For this review, take the finished solid that the model builds, in its own axes (mm). Face numbers are marked on the shaded views. A direction names the side the tool comes from. Round coordinates to 2 decimals unless told otherwise and drop trailing zeros. Order: outer loops, then holes, each group sorted by start corner. A loop starts at its lowest first (then second) coordinate and runs counter-clockwise, first axis right, second up. Notation, with made-up numbers: M 85.25,-34 L 131.25,-34 A22 cw 131.25,-19 Z; hole C 75.5,-4 d2. An arc over 180 degrees is marked long. Put each result on its own line as item: value.
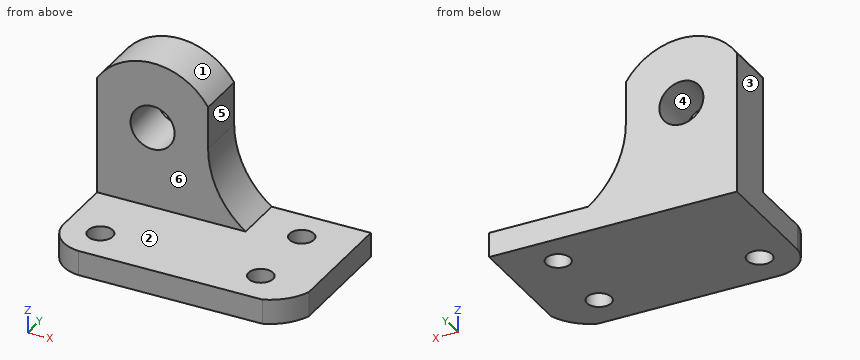
from build123d import *

# Parameters (mm, degrees)
F0_W      = 63.5
F0_H      = 38.1
F1_DEPTH  = 6.35
F3_DEPTH  = 25.4
F4_W      = 38.1
F4_H      = 12.7
F5_DEPTH  = 38.1
F7_DEPTH  = 25.4
F8_R      = 5.646791
F9_DEPTH  = 25.4
F10_R     = 3.186215
F10_R_2   = 3.13512
F10_R_3   = 3.110599
F11_DEPTH = 25.4


with BuildPart() as f1:
    # F0 (on Top) → F1 (new body)
    with BuildSketch(Plane.XY):
        with Locations((31.75, 19.05)):
            Rectangle(F0_W, F0_H)
    extrude(amount=F1_DEPTH)

    # F2 (on face) → F3 (cut)
    with BuildSketch(Plane.XY.offset(6.35)):
        with BuildLine():
            ThreePointArc((8.66646, 0), (2.760987, 2.655022), (0, 8.511703))
            Line((0, 8.511703), (0, 0))
            Line((0, 0), (8.66646, 0))
        make_face()
        with BuildLine():
            ThreePointArc((63.5, 7.892669), (60.506344, 3.058511), (55.712957, 0))
            Line((55.712957, 0), (63.5, 0))
            Line((63.5, 0), (63.5, 7.892669))
        make_face()
    extrude(amount=-F3_DEPTH, mode=Mode.SUBTRACT)

    # F4 (on face) → F5 (join)
    with BuildSketch(Plane.XY.offset(6.35)):
        with Locations((19.05, 31.75)):
            Rectangle(F4_W, F4_H)
    extrude(amount=F5_DEPTH)

    # F6 (on face) → F7 (cut)
    with BuildSketch(Plane.XZ.offset(-25.4)):
        with BuildLine():
            Line((0, 44.45), (0, 36.368184))
            ThreePointArc((0, 36.368184), (14.237756, 44.108916), (28.475512, 36.368184))
            Line((28.475512, 36.368184), (28.475512, 25.4))
            ThreePointArc((28.475512, 25.4), (31.018235, 14.728387), (38.1, 6.35))
            Line((38.1, 6.35), (38.1, 25.4))
            Line((38.1, 25.4), (38.1, 44.45))
            Line((38.1, 44.45), (0, 44.45))
        make_face()
    extrude(amount=-F7_DEPTH, mode=Mode.SUBTRACT)

    # F8 (on face) → F9 (cut)
    with BuildSketch(Plane.XZ.offset(-25.4)):
        with Locations((14.237756, 27.144589)):
            Circle(F8_R)
    extrude(amount=-F9_DEPTH, mode=Mode.SUBTRACT)

    # F10 (on face) → F11 (cut)
    with BuildSketch(Plane.XY.offset(6.35)):
        with Locations((9.307119, 9.320174)):
            Circle(F10_R)
        with Locations((50.451182, 9.320174)):
            Circle(F10_R_2)
        with Locations((50.451182, 29.249305)):
            Circle(F10_R_3)
    extrude(amount=-F11_DEPTH, mode=Mode.SUBTRACT)


solid = f1.part
(1) Draft analysis for pull direction X (two halves, no side actions). For the marked faces 3, 4, 5 and 6, state which applies: released by +X, released by -X, zero draft, split by the parting line, or undercut.
A:
face 3: released by -X
face 4: undercut
face 5: released by +X
face 6: zero draft
(2) For the marked faces 1 and 2, list the 3-axis set-ups (+Z, -Z, +X, -X, +Y, -Y) from which the entire face can be reached by the end or side of a thin tool; tool diameter is ignored.
A:
face 1: +Z, +Y, -Y
face 2: +Z, +X, -Y
(3) Add section C-C on x = 10. Give the boundary of the cut face in (y, z).
A:
outline: M 0,0 L 6.21,0 L 6.21,6.35 L 0,6.35 Z; M 12.43,0 L 38.1,0 L 38.1,23.41 L 25.4,23.41 L 25.4,6.35 L 12.43,6.35 Z; M 25.4,30.88 L 38.1,30.88 L 38.1,43.57 L 25.4,43.57 Z
(4) To check wall thickness, follow L1, parallel to Y at x = 33, z = 6.5; L2, parallel to Z at x = 50.5, y = 16; L3, parallel to X at y = 27, z = 24. State the ranges of each line that lie inside material, in increasing order.
A:
L1: y = 25.4 to 38.1
L2: z = 0 to 6.35
L3: x = 0 to 9.55, 18.93 to 28.52
(5) Add section D-D on y = 36.5. Give the boundary of the cut face in (x, z), then the cut area to 3 significant figures.
A:
outline: M 0,0 L 63.5,0 L 63.5,6.35 L 38.1,6.35 A23.67 cw 28.48,25.4 L 28.48,36.37 A16.96 ccw 0,36.37 Z; hole C 14.24,27.14 d11.29
area: 1,370 mm2
(6) Add section B-B on z = 31. Give the boundary of the cut face in (x, y).
A:
outline: M 0,25.4 L 10.11,25.4 L 10.11,38.1 L 0,38.1 Z; M 18.36,25.4 L 28.48,25.4 L 28.48,38.1 L 18.36,38.1 Z
(7) Insertion check: pin 1 Ø12 at (x, y) = (51, 18.5) entering from +Z; pin 2 Ø10 at (y, z) = (25.5, 26) entering from +X; pin 3 Ø5.5 at (y, z) = (31.5, 28.5) entering from +X. Each pin has a flat end and moves straight along its axis. Give the tip position at first contact, or say it passes through.
A:
pin 1: stops at z = 6.35
pin 2: stops at x = 28.89
pin 3: stops at x = 28.48
(8) Add section A-A on x = 17. Give the boundary of the cut face in (y, z), then the cut area to 4 significant figures.
A:
outline: M 0,0 L 38.1,0 L 38.1,22.22 L 25.4,22.22 L 25.4,6.35 L 0,6.35 Z; M 25.4,32.07 L 38.1,32.07 L 38.1,43.88 L 25.4,43.88 Z
area: 593.5 mm2
